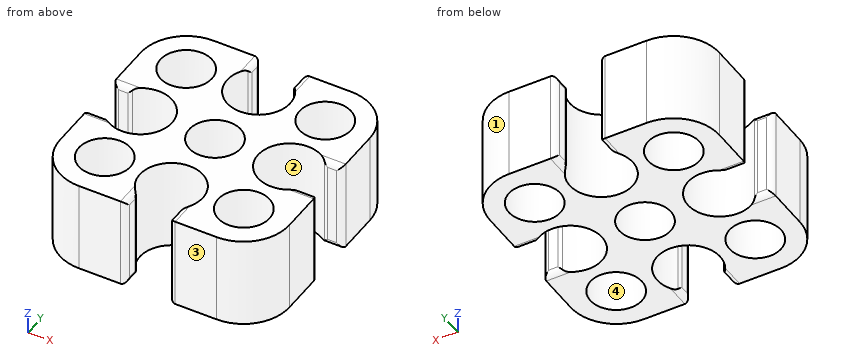
from build123d import *

# Parameters (mm, degrees)
F0_W             = 25.4
F0_H             = 25.4
F1_DEPTH         = 10.16
F2_R             = 3.4925
F3_DEPTH         = 25.4
F3_COPIES_COUNT  = 4
F5_DEPTH         = 25.4
F5_COPIES_COUNT  = 4
F7_R             = 2.8575
F8_DEPTH         = 25.4
F9_R             = 2.8575
F10_DEPTH        = 25.4
F10_COPIES_COUNT = 4
F11_R            = 5.08
F12_R            = 0.635


# Not quite as in the source:
# - a pattern or mirror of a feature is missing from the dataset's text; its kind, count and spacing are read off the source's solid


with BuildPart() as f1:
    # F0 (on Top) → F1 (new body)
    with BuildSketch(Plane.XY):
        Rectangle(F0_W, F0_H)
    extrude(amount=F1_DEPTH)

    # F2 (on face) → F3 (cut)
    with BuildSketch(Plane.XY.offset(10.16)):
        with Locations((0, -8.255)):
            Circle(F2_R)
    f3 = extrude(amount=-F3_DEPTH, mode=Mode.SUBTRACT)

    # F3_copies: F3 ×4 about axis
    f3_copies_axis = Axis((0, 0, 0), (0, 0, 1))
    for i in range(1, F3_COPIES_COUNT):
        add(f3.rotate(f3_copies_axis, i * 360 / F3_COPIES_COUNT), mode=Mode.SUBTRACT)

    # F4 (on face) → F5 (cut)
    with BuildSketch(Plane.XY.offset(10.16)):
        with BuildLine():
            Line((-2.3970724332, -10.795), (-2.3970724332, -12.7))
            Line((-2.3970724332, -12.7), (2.3970724332, -12.7))
            Line((2.3970724332, -12.7), (2.3970724332, -10.795))
            ThreePointArc((2.3970724332, -10.795), (0, -11.7475), (-2.3970724332, -10.795))
        make_face()
    f5 = extrude(amount=-F5_DEPTH, mode=Mode.SUBTRACT)

    # F5_copies: F5 ×4 about axis
    f5_copies_axis = Axis((0, 0, 0), (0, 0, 1))
    for i in range(1, F5_COPIES_COUNT):
        add(f5.rotate(f5_copies_axis, i * 360 / F5_COPIES_COUNT), mode=Mode.SUBTRACT)

    # F7 (on face) → F8 (cut)
    with BuildSketch(Plane.XY.offset(10.16)):
        Circle(F7_R)
    extrude(amount=-F8_DEPTH, mode=Mode.SUBTRACT)

    # F9 (on face) → F10 (cut)
    with BuildSketch(Plane.XY.offset(10.16)):
        with Locations((-7.7, 7.7)):
            Circle(F9_R)
    f10 = extrude(amount=-F10_DEPTH, mode=Mode.SUBTRACT)

    # F10_copies: F10 ×4 about axis
    f10_copies_axis = Axis((0, 0, 0), (0, 0, 1))
    for i in range(1, F10_COPIES_COUNT):
        add(f10.rotate(f10_copies_axis, i * 360 / F10_COPIES_COUNT), mode=Mode.SUBTRACT)

    # F11
    f11_edges = [f1.edges().sort_by_distance(p)[0] for p in [
        (-12.7, 12.7, 5.08),
        (-12.7, -12.7, 5.08),
        (12.7, -12.7, 5.08),
        (12.7, 12.7, 5.08),
    ]]
    fillet(f11_edges, radius=F11_R)

    # F12
    f12_edges = [f1.edges().sort_by_distance(p)[0] for p in [
        (2.397072, -11.7475, 10.16),
        (2.397072, -10.795, 5.08),
        (2.397072, -11.7475, 0),
        (2.397072, -12.7, 5.08),
        (-2.397072, -11.7475, 10.16),
        (-2.397072, -12.7, 5.08),
        (-2.397072, -11.7475, 0),
        (-2.397072, -10.795, 5.08),
        (11.7475, 2.397072, 0),
        (2.397072, 11.7475, 0),
        (11.7475, -2.397072, 0),
        (-2.397072, 11.7475, 0),
        (-11.7475, 2.397072, 0),
        (-11.7475, -2.397072, 0),
        (11.7475, 2.397072, 10.16),
        (2.397072, 11.7475, 10.16),
        (11.7475, -2.397072, 10.16),
        (-2.397072, 11.7475, 10.16),
        (-11.7475, 2.397072, 10.16),
        (-11.7475, -2.397072, 10.16),
        (12.7, 2.397072, 5.08),
        (10.795, 2.397072, 5.08),
        (2.397072, 12.7, 5.08),
        (10.795, -2.397072, 5.08),
        (2.397072, 10.795, 5.08),
        (12.7, -2.397072, 5.08),
        (-2.397072, 10.795, 5.08),
        (-2.397072, 12.7, 5.08),
        (-12.7, 2.397072, 5.08),
        (-10.795, 2.397072, 5.08),
        (-10.795, -2.397072, 5.08),
        (-12.7, -2.397072, 5.08),
    ]]
    fillet(f12_edges, radius=F12_R)


solid = f1.part
Can you work these out from the model? Positions are in its coordinate system, mm. Face numbers are marked on the shaded views. Give positions to 0.01 mm unless a question says otherwise; leave off trailing zeros. Loops run counter-clockwise (first coordinate to the right, second up) from the corner with the lowest first, then second, coordinate; pieces in that order, holes last. Notation, with made-up numbers: (-35.5, 30.5) - (-13.5, 30.5) arc R30 cw to (-13.5, 67.5) - close; hole circle Ø10 at (29.25, -3.5). An arc over 180 degrees is marked (long way). Answer as a JSON object with one key per item and string values.
Q1. Imagine slicing it at D-D on z = 2.5. Give the number of separate pieces and of enclosed holes in the cut face, plus the area to 3 significant figures.
Geometry says:
{"separate pieces": "1", "enclosed holes": "5", "area": "317 mm²"}
Q2. Imagine slicing it at A-A on x = 0. Write out the boundary of the cut face in (y, z).
Geometry says:
{"outline": "(-4.76, 0) - (-2.86, 0) - (-2.86, 10.16) - (-4.76, 10.16) - close; (2.86, 0) - (4.76, 0) - (4.76, 10.16) - (2.86, 10.16) - close"}
Q3. If we mould it in two halves opening along X, with no side actions, what happens to the marked faces 1, 2, 3 and 4? For each: pulls with the +X half, pulls with the -X half, needs draft (parallel to the pull), parting line crosses it, or undercut.
Geometry says:
{"face 1": "pulls with the +X half", "face 2": "undercut", "face 3": "needs draft", "face 4": "undercut"}
Q4. Imagine slicing it at C-C on x = -7. Write out the boundary of the cut face in (y, z).
Geometry says:
{"outline": "(-12.7, 0) - (-10.47, 0) - (-10.47, 10.16) - (-12.7, 10.16) - close; (-4.93, 0) - (-3.26, 0) - (-3.26, 10.16) - (-4.93, 10.16) - close; (3.26, 0) - (4.93, 0) - (4.93, 10.16) - (3.26, 10.16) - close; (10.47, 0) - (12.7, 0) - (12.7, 10.16) - (10.47, 10.16) - close"}
Q5. Imagine slicing it at B-B on y = -9.25. Write out the boundary of the cut face in (x, z).
Geometry says:
{"outline": "(-12.43, 0) - (-10.1, 0) - (-10.1, 10.16) - (-12.43, 10.16) - close; (-5.3, 0) - (-3.35, 0) - (-3.35, 10.16) - (-5.3, 10.16) - close; (3.35, 0) - (5.3, 0) - (5.3, 10.16) - (3.35, 10.16) - close; (10.1, 0) - (12.43, 0) - (12.43, 10.16) - (10.1, 10.16) - close"}
Q6. Will these pins go through, and if not, where does the flat tip stop? P1, Ø0.8, axis at y = -11.5, z = 4, coming from the -X side; P2, Ø0.5, axis at y = -12, z = 5.5, coming from the +X side; P3, Ø0.5, axis at y = 11.5, z = 4.5, coming from the +X side.
Geometry says:
{"P1": "x = -11.32", "P2": "x = 10.58", "P3": "x = 11.17"}
Q7. If I drill on L1, parallel to Y at x = 0, z = 3.25; L2, parallel to Y at x = 3, z = 7; L3, parallel to Y at x = -7.75, z = 8, over which ranges is the centre line in solid material (lowest first)?
Geometry says:
{"L1": "-4.76 to -2.86, 2.86 to 4.76", "L2": "-12.7 to -10.04, -6.47 to 6.47, 10.04 to 12.7", "L3": "-12.7 to -10.56, -4.84 to -3.46, 3.46 to 4.84, 10.56 to 12.7"}
